The model under review builds one solid part; all positions refer to its coordinate system, in mm. A direction names the side the tool comes from. Coordinates: 2 decimals unless noted, no trailing zeros. Order: outer loops, then holes, each group sorted by start corner. A loop starts at its lowest first (then second) coordinate and runs counter-clockwise, first axis right, second up. Notation, with made-up numbers: (10.5, -26) -> (57.5, -26) arc R33 ccw to (57.5, 5) -> close; hole circle Ø3 at (61.5, -30). An arc over 180 degrees is marked (long way). Use CSV: the item, a comma, the result in double quotes. Start each with the question number.
```python
from build123d import *

# Parameters (mm, degrees)
SKETCH1_W           = 100
SKETCH1_H           = 80
BOSS_EXTRUDE1_DEPTH = 4


with BuildPart() as part:
    # Sketch1 → Boss-Extrude1 (new body)
    with BuildSketch(Plane.XY):
        with Locations((50, 40)):
            Rectangle(SKETCH1_W, SKETCH1_H)
        with BuildLine():
            Line((12.55, 68), (12.55, 48))
            ThreePointArc((12.55, 48), (10, 45.45), (7.45, 48))
            Line((7.45, 48), (7.45, 68))
            ThreePointArc((7.45, 68), (10, 70.55), (12.55, 68))
        make_face(mode=Mode.SUBTRACT)
        with BuildLine():
            Line((12.55, 32), (12.55, 12))
            ThreePointArc((12.55, 12), (10, 9.45), (7.45, 12))
            Line((7.45, 12), (7.45, 32))
            ThreePointArc((7.45, 32), (10, 34.55), (12.55, 32))
        make_face(mode=Mode.SUBTRACT)
        with BuildLine():
            Line((92.55, 68), (92.55, 48))
            ThreePointArc((92.55, 48), (90, 45.45), (87.45, 48))
            Line((87.45, 48), (87.45, 68))
            ThreePointArc((87.45, 68), (90, 70.55), (92.55, 68))
        make_face(mode=Mode.SUBTRACT)
        with BuildLine():
            Line((92.55, 32), (92.55, 12))
            ThreePointArc((92.55, 12), (90, 9.45), (87.45, 12))
            Line((87.45, 12), (87.45, 32))
            ThreePointArc((87.45, 32), (90, 34.55), (92.55, 32))
        make_face(mode=Mode.SUBTRACT)
    extrude(amount=BOSS_EXTRUDE1_DEPTH)


solid = part.part
```
Q1. Add section A-A, the plane z = 2.35. State the section outline as (x, y) points.
Q2. Draft analysis for pull direction X (two halves, no side actions). For faces 1 (the cylindrical face through (9.94, 70.55, 1.97)), 2 (the flat face through (0, 39, 2)), 3 (the flat face through (49, 41, 0)), state which applies: +X half, -X half, draft (parallel to the pull), parting line (faces both ways), or undercut.
Q3. Add section B-B, the plane x = 90. State the section outline as (y, z) points.
Q4. Add section C-C, the plane y = 10.5. State the section outline as (x, z) points.
Q5. To check wall thickness, follow probe 1 along X at (y, z) = (54, 1.9); probe 2 along Y at (x, z) = (90, 0.55). State the ranges of each line that lie inside material, in increasing order.
Q6. For faces 4 (the cylindrical face through (10.06, 45.45, 1.97)), 5 (the flat face through (49, 41, 4)), list the 3-axis set-ups (+Z, -Z, +X, -X, +Y, -Y) from which the entire face can be reached by the end or side of a thin tool; tool diameter is ignored.
Answer block:
1,outline,"(0, 0) -> (100, 0) -> (100, 80) -> (0, 80) -> close; hole (7.45, 12) arc R2.55 ccw to (12.55, 12) -> (12.55, 32) arc R2.55 ccw to (7.45, 32) -> close; hole (7.45, 48) arc R2.55 ccw to (12.55, 48) -> (12.55, 68) arc R2.55 ccw to (7.45, 68) -> close; hole (87.45, 12) arc R2.55 ccw to (92.55, 12) -> (92.55, 32) arc R2.55 ccw to (87.45, 32) -> close; hole (87.45, 48) arc R2.55 ccw to (92.55, 48) -> (92.55, 68) arc R2.55 ccw to (87.45, 68) -> close"
2,face 1,"undercut"
2,face 2,"-X half"
2,face 3,"draft"
3,outline,"(0, 0) -> (9.45, 0) -> (9.45, 4) -> (0, 4) -> close; (34.55, 0) -> (45.45, 0) -> (45.45, 4) -> (34.55, 4) -> close; (70.55, 0) -> (80, 0) -> (80, 4) -> (70.55, 4) -> close"
4,outline,"(0, 0) -> (7.94, 0) -> (7.94, 4) -> (0, 4) -> close; (12.06, 0) -> (87.94, 0) -> (87.94, 4) -> (12.06, 4) -> close; (92.06, 0) -> (100, 0) -> (100, 4) -> (92.06, 4) -> close"
5,probe 1,"x = 0 to 7.45, 12.55 to 87.45, 92.55 to 100"
5,probe 2,"y = 0 to 9.45, 34.55 to 45.45, 70.55 to 80"
6,face 4,"+Z, -Z"
6,face 5,"+Z, +X, -X, +Y, -Y"
